```python
from build123d import *

# Parameters (mm, degrees)
SKETCH1_R           = 22.5
SKETCH1_R_2         = 11
SKETCH1_R_3         = 2.25
BOSS_EXTRUDE1_DEPTH = 8
CHAMFER1_SIZE       = 1


with BuildPart() as part:
    # Sketch1 → Boss-Extrude1 (new body)
    with BuildSketch(Plane(origin=(0, 0, 0), x_dir=(1, 0, 0), z_dir=(0, 1, 0))):
        with Locations(Location((0, 0, 0), (0, 0, 270))):
            Circle(SKETCH1_R)
        with Locations(Location((0, 0, 0), (0, 0, 270))):
            Circle(SKETCH1_R_2, mode=Mode.SUBTRACT)
        with Locations(Location((-15, 0, 0), (0, 0, 270))):
            Circle(SKETCH1_R_3, mode=Mode.SUBTRACT)
        with Locations(Location((15, 0, 0), (0, 0, 270))):
            Circle(SKETCH1_R_3, mode=Mode.SUBTRACT)
        with Locations(Location((0, -15, 0), (0, 0, 270))):
            Circle(SKETCH1_R_3, mode=Mode.SUBTRACT)
        with Locations(Location((0, 15, 0), (0, 0, 270))):
            Circle(SKETCH1_R_3, mode=Mode.SUBTRACT)
    extrude(amount=BOSS_EXTRUDE1_DEPTH)

    # Chamfer1
    # the kernel refuses this chamfer: 1 mm, written as the material it takes off along each edge
    with BuildSketch(Plane(origin=(15, 0, 0), x_dir=(0, 0, 1), z_dir=(-1, 0, 0))) as chamfer1_piece_1:
        Polygon((2.25, CHAMFER1_SIZE), (2.25 + CHAMFER1_SIZE, 0), (2.25, 0), align=None)
    revolve(axis=Axis((15, 0, 0), (0, 1, 0)), mode=Mode.SUBTRACT)
    with BuildSketch(Plane(origin=(15, 8, 0), x_dir=(0, 0, 1), z_dir=(-1, 0, 0))) as chamfer1_piece_2:
        Polygon((2.25, -CHAMFER1_SIZE), (2.25 + CHAMFER1_SIZE, 0), (2.25, 0), align=None)
    revolve(axis=Axis((15, 8, 0), (0, 1, 0)), mode=Mode.SUBTRACT)
    with BuildSketch(Plane(origin=(0, 0, -15), x_dir=(0, 0, 1), z_dir=(-1, 0, 0))) as chamfer1_piece_3:
        Polygon((2.25, CHAMFER1_SIZE), (2.25 + CHAMFER1_SIZE, 0), (2.25, 0), align=None)
    revolve(axis=Axis((0, 0, -15), (0, 1, 0)), mode=Mode.SUBTRACT)
    with BuildSketch(Plane(origin=(0, 8, -15), x_dir=(0, 0, 1), z_dir=(-1, 0, 0))) as chamfer1_piece_4:
        Polygon((2.25, -CHAMFER1_SIZE), (2.25 + CHAMFER1_SIZE, 0), (2.25, 0), align=None)
    revolve(axis=Axis((0, 8, -15), (0, 1, 0)), mode=Mode.SUBTRACT)
    with BuildSketch(Plane(origin=(0, 0, 0), x_dir=(0, 0, 1), z_dir=(-1, 0, 0))) as chamfer1_piece_5:
        Polygon((22.5, CHAMFER1_SIZE), (22.5 - CHAMFER1_SIZE, 0), (22.5, 0), align=None)
    revolve(axis=Axis((0, 0, 0), (0, 1, 0)), mode=Mode.SUBTRACT)
    with BuildSketch(Plane(origin=(-15, 0, 0), x_dir=(0, 0, 1), z_dir=(-1, 0, 0))) as chamfer1_piece_6:
        Polygon((2.25, CHAMFER1_SIZE), (2.25 + CHAMFER1_SIZE, 0), (2.25, 0), align=None)
    revolve(axis=Axis((-15, 0, 0), (0, 1, 0)), mode=Mode.SUBTRACT)
    with BuildSketch(Plane(origin=(-15, 8, 0), x_dir=(0, 0, 1), z_dir=(-1, 0, 0))) as chamfer1_piece_7:
        Polygon((2.25, -CHAMFER1_SIZE), (2.25 + CHAMFER1_SIZE, 0), (2.25, 0), align=None)
    revolve(axis=Axis((-15, 8, 0), (0, 1, 0)), mode=Mode.SUBTRACT)
    with BuildSketch(Plane(origin=(0, 8, 0), x_dir=(0, 0, 1), z_dir=(-1, 0, 0))) as chamfer1_piece_8:
        Polygon((22.5, -CHAMFER1_SIZE), (22.5 - CHAMFER1_SIZE, 0), (22.5, 0), align=None)
    revolve(axis=Axis((0, 8, 0), (0, 1, 0)), mode=Mode.SUBTRACT)
    with BuildSketch(Plane(origin=(0, 0, 0), x_dir=(0, 0, 1), z_dir=(-1, 0, 0))) as chamfer1_piece_9:
        Polygon((11, CHAMFER1_SIZE), (11 + CHAMFER1_SIZE, 0), (11, 0), align=None)
    revolve(axis=Axis((0, 0, 0), (0, 1, 0)), mode=Mode.SUBTRACT)
    with BuildSketch(Plane(origin=(0, 8, 0), x_dir=(0, 0, 1), z_dir=(-1, 0, 0))) as chamfer1_piece_10:
        Polygon((11, -CHAMFER1_SIZE), (11 + CHAMFER1_SIZE, 0), (11, 0), align=None)
    revolve(axis=Axis((0, 8, 0), (0, 1, 0)), mode=Mode.SUBTRACT)
    with BuildSketch(Plane(origin=(0, 0, 15), x_dir=(0, 0, 1), z_dir=(-1, 0, 0))) as chamfer1_piece_11:
        Polygon((2.25, CHAMFER1_SIZE), (2.25 + CHAMFER1_SIZE, 0), (2.25, 0), align=None)
    revolve(axis=Axis((0, 0, 15), (0, 1, 0)), mode=Mode.SUBTRACT)
    with BuildSketch(Plane(origin=(0, 8, 15), x_dir=(0, 0, 1), z_dir=(-1, 0, 0))) as chamfer1_piece_12:
        Polygon((2.25, -CHAMFER1_SIZE), (2.25 + CHAMFER1_SIZE, 0), (2.25, 0), align=None)
    revolve(axis=Axis((0, 8, 15), (0, 1, 0)), mode=Mode.SUBTRACT)


solid = part.part
```
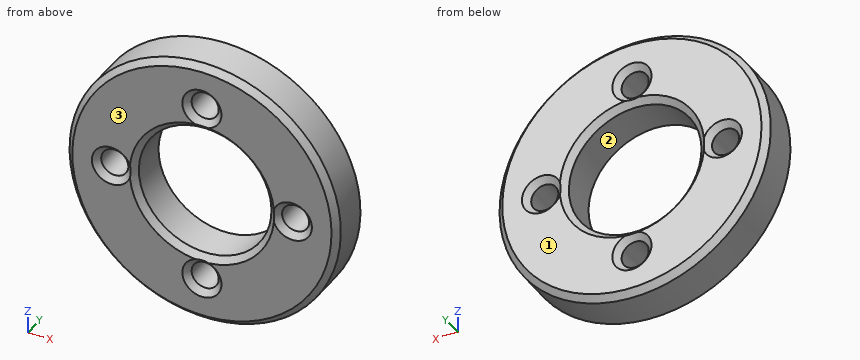
Input: part model. Units: mm. Frame: model coordinates. Face numbers are marked on the shaded views. Give positions to 0.01 mm unless a question says otherwise; leave off trailing zeros. Loops run counter-clockwise (first coordinate to the right, second up) from the corner with the lowest first, then second, coordinate; pieces in that order, holes last.
1) Section query A-A on y = 2.75. Return the cut outline in (x, z), and give its area (3 significant figures).
A:
outline: circle Ø45 at (0, 0); hole circle Ø4.5 at (-15, 0); hole circle Ø22 at (0, 0); hole circle Ø4.5 at (0, -15); hole circle Ø4.5 at (0, 15); hole circle Ø4.5 at (15, 0)
area: 1,150 mm2
2) Line query: L1, parallel to X at y = 2.35, z = 0; L2, parallel to Z at x = -14.5, y = 7.25; L3, parallel to X at y = 6.25, z = -9. Output: solid intervals per line, ascending.
A:
L1: x = -22.5 to -17.25, -12.75 to -11, 11 to 12.75, 17.25 to 22.5
L2: z = -16.88 to -2.45, 2.45 to 16.88
L3: x = -20.62 to -6.32, 6.32 to 20.62
3) Contact query for flat-ended pins moving along their axis: pin 1 (10 mm diameter, centred on x = 11.5, z = -3, fed in from +Y); pin 2 (3 mm diameter, centred on y = 6, z = 16.5, fed in from -X); pin 3 (5 mm diameter, centred on x = -15, z = 0, fed in from +Y); pin 4 (4 mm diameter, centred on y = 7, z = 0.5, fed in from +X). Output: stop coordinate, or through.
A:
pin 1: stops at y = 8
pin 2: stops at x = -16.77
pin 3: stops at y = 7.25
pin 4: stops at x = 22.5
4) Section query B-B on x = 0. Return the cut outline in (y, z) (3 decimals), and give its area (3 significant figures).
A:
outline: (0, -21.5) - (1, -22.5) - (7, -22.5) - (8, -21.5) - (8, -18.25) - (7, -17.25) - (1, -17.25) - (0, -18.25) - close; (0, 18.25) - (1, 17.25) - (7, 17.25) - (8, 18.25) - (8, 21.5) - (7, 22.5) - (1, 22.5) - (0, 21.5) - close; (0.125, -11.875) - (1, -12.75) - (7, -12.75) - (7.875, -11.875) - (7, -11) - (1, -11) - close; (0.125, 11.875) - (1, 11) - (7, 11) - (7.875, 11.875) - (7, 12.75) - (1, 12.75) - close
area: 104 mm2
5) Mould query, pull axis Y, two halves, no side actions, for the marked faces 1, 2 and 3. Classes: released by +Y, released by -Y, zero draft, split by the parting line, or undercut.
A:
face 1: released by +Y
face 2: zero draft
face 3: released by -Y
